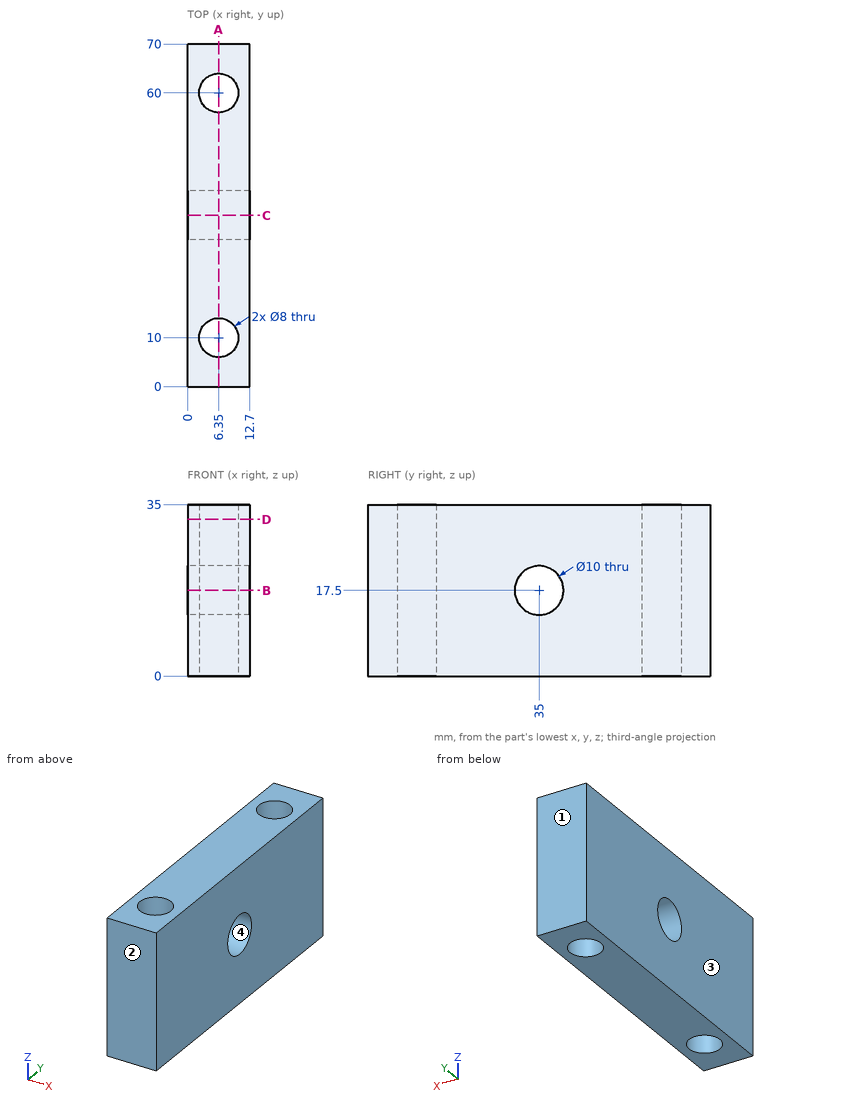
Answer from the drawing. Dimensions are ordinates in mm from the lowest x, y and z of the part. Coordinates: 2 decimals unless noted, no trailing zeros. Loops run counter-clockwise (first coordinate to the right, second up) from the corner with the lowest first, then second, coordinate; pieces in that order, holes last. Notation, with made-up numbers: (3, -30.5) -> (18, -30.5) arc R16 ccw to (18, -0.5) -> close; hole circle Ø6 at (83.25, 68.25). An arc over 180 degrees is marked (long way). Answer in a Markdown table with one row per item.
Item 1: Straight lines are drawn through the part: line 1 along Y through (x, z) = (6.35, 25); line 2 along Y through (x, z) = (7.5, 25); line 3 along Y through (x, z) = (8.25, 21). For each, find the intervals that lie inside material, in ascending order. Write a range as [from, to].
Returned:
| item | result |
|---|---|
| line 1 | y = [0, 6], [14, 56], [64, 70] |
| line 2 | y = [0, 6.17], [13.83, 56.17], [63.83, 70] |
| line 3 | y = [0, 6.48], [13.52, 31.43], [38.57, 56.48], [63.52, 70] |
Item 2: A cutting plane is placed at C-C on y = 35. Determine the outline of the cut face in (x, z).
Returned:
| item | result |
|---|---|
| outline | (0, 0) -> (12.7, 0) -> (12.7, 12.5) -> (0, 12.5) -> close; (0, 22.5) -> (12.7, 22.5) -> (12.7, 35) -> (0, 35) -> close |
Item 3: A cutting plane is placed at D-D on z = 32. Determine the outline of the cut face in (x, y).
Returned:
| item | result |
|---|---|
| outline | (0, 0) -> (12.7, 0) -> (12.7, 70) -> (0, 70) -> close; hole circle Ø8 at (6.35, 10); hole circle Ø8 at (6.35, 60) |
Item 4: A cutting plane is placed at B-B on z = 17.5. Determine the outline of the cut face in (x, y), plus the area to 3 significant figures.
Returned:
| item | result |
|---|---|
| outline | (0, 0) -> (12.7, 0) -> (12.7, 30) -> (0, 30) -> close; (0, 40) -> (12.7, 40) -> (12.7, 70) -> (0, 70) -> close; hole circle Ø8 at (6.35, 10); hole circle Ø8 at (6.35, 60) |
| area | 661 mm^2 |
Item 5: A cutting plane is placed at A-A on x = 6.35. Determine the outline of the cut face in (y, z), plus the area to 3 significant figures.
Returned:
| item | result |
|---|---|
| outline | (0, 0) -> (6, 0) -> (6, 35) -> (0, 35) -> close; (14, 0) -> (56, 0) -> (56, 35) -> (14, 35) -> close; (64, 0) -> (70, 0) -> (70, 35) -> (64, 35) -> close; hole circle Ø10 at (35, 17.5) |
| area | 1,810 mm^2 |
Item 6: For a pull along Y with two mould halves and no side action, classify the marked faces 1, 2, 3 and 4 as released by +Y, released by -Y, zero draft, split by the parting line, or undercut.
Returned:
| item | result |
|---|---|
| face 1 | released by +Y |
| face 2 | released by -Y |
| face 3 | zero draft |
| face 4 | undercut |
